from build123d import *

# Parameters (mm, degrees)
SKETCH_1_R      = 23
EXTRUDE_1_DEPTH = 4


with BuildPart() as part:
    # 草图1 → 凸台-拉伸1 (new body)
    with BuildSketch(Plane.XY):
        Polygon((37.5, 50), (-37.5, 50), (-43.5, 50), (-43.5, -50), (-43.5, -150), (-37.5, -150), (37.5, -150), (43.5, -150), (43.5, -50), (43.5, 50), align=None)
        with Locations((0, -53)):
            Circle(SKETCH_1_R, mode=Mode.SUBTRACT)
    extrude(amount=EXTRUDE_1_DEPTH)


solid = part.part
For this review, take the finished solid that the model builds, in its own axes (mm). Give positions to 0.01 mm unless a question says otherwise; leave off trailing zeros. Order: outer loops, then holes, each group sorted by start corner. A loop starts at its lowest first (then second) coordinate and runs counter-clockwise, first axis right, second up. Notation, with made-up numbers: M -20,-26.75 L 7,-26.75 A30 cw 7,6.25 Z; hole C 25,11 d8. An arc over 180 degrees is marked long. Answer in a Markdown table with one row per item. Add a question column.
(1) Consider section A-A on x = 0. State the section outline as (y, z) points, and give its area (3 significant figures).
(2) Consider section C-C on z = 2.65. State the section outline as (x, y) points.
(3) Mouldability with a two-part tool opening along Y and no side actions: class faces 1 (the face through (-2.994, -30.196, 1.972)), 2 (the face through (-1, -26, 4)), 3 (the face through (-1, -150, 2)), 4 (the face through (1, 50, 2)) as +Y half, -Y half, draft (parallel to the pull), parting line (faces both ways), or undercut.
(4) Wall thickness on probe 1 along Y at (x, z) = (0, 2.8); probe 2 along Y at (x, z) = (3.5, 2.3); probe 3 along X at (y, z) = (-39, 0.25): over which ranges is each line inside the solid? List them lowest first. Write a range as [from, to].
(5) Consider section B-B on y = -53. State the section outline as (x, z) points.
Evaluation:
| question | item | result |
|---|---|---|
| 1 | outline | M -150,0 L -76,0 L -76,4 L -150,4 Z; M -30,0 L 50,0 L 50,4 L -30,4 Z |
| 1 | area | 616 mm^2 |
| 2 | outline | M -43.5,-150 L 43.5,-150 L 43.5,50 L -43.5,50 Z; hole C 0,-53 d46 |
| 3 | face 1 | undercut |
| 3 | face 2 | draft |
| 3 | face 3 | -Y half |
| 3 | face 4 | +Y half |
| 4 | probe 1 | y = [-150, -76], [-30, 50] |
| 4 | probe 2 | y = [-150, -75.73], [-30.27, 50] |
| 4 | probe 3 | x = [-43.5, -18.25], [18.25, 43.5] |
| 5 | outline | M -43.5,0 L -23,0 L -23,4 L -43.5,4 Z; M 23,0 L 43.5,0 L 43.5,4 L 23,4 Z |
